```python
from build123d import *

# Parameters (mm, degrees)
F0_W     = 914.4
F0_H     = 457.2
F1_DEPTH = 50.8
F3_DEPTH = 838.2


with BuildPart() as f1:
    # F0 (on Top) → F1 (new body)
    with BuildSketch(Plane.XY):
        with Locations((457.2, -228.6)):
            Rectangle(F0_W, F0_H)
    extrude(amount=F1_DEPTH)

    # F2 (on face) → F3 (join)
    with BuildSketch(Plane(origin=(0, 0, 0), x_dir=(1, 0, 0), z_dir=(0, 0, -1))):
        with BuildLine():
            ThreePointArc((914.4, 431.8), (906.960512, 449.760512), (889, 457.2))
            ThreePointArc((889, 457.2), (871.039488, 449.760512), (863.6, 431.8))
            ThreePointArc((863.6, 431.8), (871.039488, 413.839488), (889, 406.4))
            ThreePointArc((889, 406.4), (906.960512, 413.839488), (914.4, 431.8))
        make_face()
        with BuildLine():
            ThreePointArc((914.4, 25.4), (906.960512, 43.360512), (889, 50.8))
            ThreePointArc((889, 50.8), (871.039488, 43.360512), (863.6, 25.4))
            ThreePointArc((863.6, 25.4), (871.039488, 7.439488), (889, 0))
            ThreePointArc((889, 0), (906.960512, 7.439488), (914.4, 25.4))
        make_face()
        with BuildLine():
            ThreePointArc((50.8, 25.4), (43.360512, 43.360512), (25.4, 50.8))
            ThreePointArc((25.4, 50.8), (7.439488, 43.360512), (0, 25.4))
            ThreePointArc((0, 25.4), (7.439488, 7.439488), (25.4, 0))
            ThreePointArc((25.4, 0), (43.360512, 7.439488), (50.8, 25.4))
        make_face()
        with BuildLine():
            ThreePointArc((50.8, 431.8), (43.360512, 449.760512), (25.4, 457.2))
            ThreePointArc((25.4, 457.2), (7.439488, 449.760512), (0, 431.8))
            ThreePointArc((0, 431.8), (7.439488, 413.839488), (25.4, 406.4))
            ThreePointArc((25.4, 406.4), (43.360512, 413.839488), (50.8, 431.8))
        make_face()
    extrude(amount=F3_DEPTH)


solid = f1.part
```
Read the model definition and answer for the solid it produces. Units are mm, in the model's axes. A direction names the side the tool comes from. Give positions to 0.01 mm unless a question says otherwise; leave off trailing zeros. Order: outer loops, then holes, each group sorted by start corner. A loop starts at its lowest first (then second) coordinate and runs counter-clockwise, first axis right, second up. Notation, with made-up numbers: (17, 59) -> (46, 59) arc R20 ccw to (46, 82) -> close; hole circle Ø8 at (14.25, 31.25). An arc over 180 degrees is marked (long way). One line per item, written item: value. Start each with the question number.
(1) The part is cut by section C-C (y = -323). Determine the outline of the cut face in (x, z), and give its area (3 significant figures).
(2) The part is cut by section A-A (z = -294). Determine the outline of the cut face in (x, y), and give its area (3 significant figures).
(3) A tool of negligible diameter and unlimited length cuts with its end or side. For faces 1 (the flat face through (908, -5, 0)), 2 (the flat face through (0, -232, 25)), 3 (the flat face through (5, -451, 0)), 4 (the flat face through (5, -6, 0)), 5 (the flat face through (909, -452, 0)), from which of +Z, -Z, +X, -X, +Y, -Y can it reach the whole face along a straight path? Write none if from no direction.
(4) The part is cut by section B-B (x = 205.5). Determine the outline of the cut face in (y, z).
(5) Straight lines are drawn through the part: L1, parallel to Z at x = 393.5, y = -203; L2, parallel to Y at x = 44, z = -391. For each, find the intervals that lie inside material, in ascending order.
(6) For a pull along X with two mould halves and no side action, classify faces 6 (the flat face through (914.4, -232, 25)), 7 (the flat face through (451, -225, 0)), 8 (the flat face through (451, 0, 25)) as released by +X, released by -X, zero draft, split by the parting line, or undercut.
Taken from the geometry:
1. outline: (0, 0) -> (914.4, 0) -> (914.4, 50.8) -> (0, 50.8) -> close
1. area: 46,500 mm^2
2. outline: (0, -431.8) arc R25.4 ccw to (25.4, -457.2) arc R25.4 ccw to (50.8, -431.8) arc R25.4 ccw to (25.4, -406.4) arc R25.4 ccw to start; (0, -25.4) arc R25.4 ccw to (25.4, -50.8) arc R25.4 ccw to (50.8, -25.4) arc R25.4 ccw to (25.4, 0) arc R25.4 ccw to start; (863.6, -431.8) arc R25.4 ccw to (889, -457.2) arc R25.4 ccw to (914.4, -431.8) arc R25.4 ccw to (889, -406.4) arc R25.4 ccw to start; (863.6, -25.4) arc R25.4 ccw to (889, -50.8) arc R25.4 ccw to (914.4, -25.4) arc R25.4 ccw to (889, 0) arc R25.4 ccw to start
2. area: 8,110 mm^2
3. face 1: -Z, +X, +Y
3. face 2: +Z, -Z, -X, +Y, -Y
3. face 3: -Z, -X, -Y
3. face 4: -Z, -X, +Y
3. face 5: -Z, +X, -Y
4. outline: (-457.2, 0) -> (0, 0) -> (0, 50.8) -> (-457.2, 50.8) -> close
5. L1: 0 to 50.8
5. L2: -449.1 to -414.5, -42.7 to -8.1
6. face 6: released by +X
6. face 7: undercut
6. face 8: zero draft
